Check sheet for the modelled part. Datum: model origin and axes. Units: mm. A direction names the side the tool comes from. Give positions to 0.01 mm unless a question says otherwise; leave off trailing zeros. Loops run counter-clockwise (first coordinate to the right, second up) from the corner with the lowest first, then second, coordinate; pieces in that order, holes last. Notation, with made-up numbers: (45.5, -23.75) - (73.5, -23.75) arc R15 cw to (73.5, 3.25) - close; hole circle Ø3 at (60.25, -30). An arc over 180 degrees is marked (long way). Use CSV: the item, a comma, the result in double quotes.
from build123d import *

# Parameters (mm, degrees)
F0_R     = 1
F0_R_2   = 1.5
F1_DEPTH = 0.5
F2_R     = 1
F2_R_2   = 2.2
F3_DEPTH = 1
F4_SIZE  = 0.99999
F5_R     = 1
F6_DEPTH = 1
F8_DEPTH = 1


# Not quite as in the source:
# - a fillet or chamfer is up to 0.001 mm smaller than in the source, because OpenCascade refuses the exact size


with BuildPart() as f1:
    # F0 (on Top) → F1 (new body)
    with BuildSketch(Plane.XY):
        with BuildLine():
            Line((-6.2, -5.1), (6.2, -5.1))
            ThreePointArc((6.2, -5.1), (8.3213203436, -4.2213203436), (9.2, -2.1))
            Line((9.2, -2.1), (9.2, 2.1))
            ThreePointArc((9.2, 2.1), (8.3213203436, 4.2213203436), (6.2, 5.1))
            Line((6.2, 5.1), (-6.2, 5.1))
            ThreePointArc((-6.2, 5.1), (-8.3213203436, 4.2213203436), (-9.2, 2.1))
            Line((-9.2, 2.1), (-9.2, -2.1))
            ThreePointArc((-9.2, -2.1), (-8.3213203436, -4.2213203436), (-6.2, -5.1))
        make_face()
        with Locations((-5.7, -2.2)):
            Circle(F0_R, mode=Mode.SUBTRACT)
        with Locations((5.7, -2.2)):
            Circle(F0_R, mode=Mode.SUBTRACT)
        with Locations((-5.7, 2.2)):
            Circle(F0_R, mode=Mode.SUBTRACT)
        Circle(F0_R_2, mode=Mode.SUBTRACT)
        with Locations((5.7, 2.2)):
            Circle(F0_R, mode=Mode.SUBTRACT)
    extrude(amount=F1_DEPTH)

    # F2 (on face) → F3 (join)
    with BuildSketch(Plane.XY.offset(0.5)):
        with BuildLine():
            ThreePointArc((-6.2, 5.1), (-8.3213203436, 4.2213203436), (-9.2, 2.1))
            Line((-9.2, 2.1), (-9.2, -2.1))
            ThreePointArc((-9.2, -2.1), (-8.3213203436, -4.2213203436), (-6.2, -5.1))
            Line((-6.2, -5.1), (6.2, -5.1))
            ThreePointArc((6.2, -5.1), (8.3213203436, -4.2213203436), (9.2, -2.1))
            Line((9.2, -2.1), (9.2, 2.1))
            ThreePointArc((9.2, 2.1), (8.3213203436, 4.2213203436), (6.2, 5.1))
            Line((6.2, 5.1), (-6.2, 5.1))
        make_face()
        with Locations((-5.7, -2.2)):
            Circle(F2_R, mode=Mode.SUBTRACT)
        Circle(F2_R_2, mode=Mode.SUBTRACT)
        with Locations((5.7, -2.2)):
            Circle(F2_R, mode=Mode.SUBTRACT)
        with Locations((-5.7, 2.2)):
            Circle(F2_R, mode=Mode.SUBTRACT)
        with Locations((5.7, 2.2)):
            Circle(F2_R, mode=Mode.SUBTRACT)
    extrude(amount=F3_DEPTH)

    # F4 (size 1 in the source; OpenCascade refuses exactly that, so slightly less here)
    f4_edges = [f1.edges().sort_by_distance(p)[0] for p in [
        (-2.2, 0, 1.5),
    ]]
    chamfer(f4_edges, length=F4_SIZE)

    # F5 (on face) → F6 (join)
    with BuildSketch(Plane.XY.offset(1.5)):
        with BuildLine():
            Line((6.2, 5.1), (-6.2, 5.1))
            ThreePointArc((-6.2, 5.1), (-8.3213203436, 4.2213203436), (-9.2, 2.1))
            Line((-9.2, 2.1), (-9.2, -2.1))
            ThreePointArc((-9.2, -2.1), (-8.3213203436, -4.2213203436), (-6.2, -5.1))
            Line((-6.2, -5.1), (6.2, -5.1))
            ThreePointArc((6.2, -5.1), (8.3213203436, -4.2213203436), (9.2, -2.1))
            Line((9.2, -2.1), (9.2, 2.1))
            ThreePointArc((9.2, 2.1), (8.3213203436, 4.2213203436), (6.2, 5.1))
        make_face()
        with Locations((-5.7, -2.2)):
            Circle(F5_R, mode=Mode.SUBTRACT)
        with BuildLine():
            ThreePointArc((3.5, -3), (3.3535533906, -3.3535533906), (3, -3.5))
            Line((3, -3.5), (-3, -3.5))
            ThreePointArc((-3, -3.5), (-3.3535533906, -3.3535533906), (-3.5, -3))
            Line((-3.5, -3), (-3.5, 3))
            ThreePointArc((-3.5, 3), (-3.3535533906, 3.3535533906), (-3, 3.5))
            Line((-3, 3.5), (3, 3.5))
            ThreePointArc((3, 3.5), (3.3535533906, 3.3535533906), (3.5, 3))
            Line((3.5, 3), (3.5, -3))
        make_face(mode=Mode.SUBTRACT)
        with Locations((5.7, -2.2)):
            Circle(F5_R, mode=Mode.SUBTRACT)
        with Locations((-5.7, 2.2)):
            Circle(F5_R, mode=Mode.SUBTRACT)
        with Locations((5.7, 2.2)):
            Circle(F5_R, mode=Mode.SUBTRACT)
    extrude(amount=F6_DEPTH)

    # F7 (on face) → F8 (join)
    with BuildSketch(Plane.XY.offset(2.5)):
        with BuildLine():
            ThreePointArc((6.2, -5.1), (8.3213203436, -4.2213203436), (9.2, -2.1))
            Line((9.2, -2.1), (9.2, 2.1))
            ThreePointArc((9.2, 2.1), (8.3213203436, 4.2213203436), (6.2, 5.1))
            Line((6.2, 5.1), (-6.2, 5.1))
            ThreePointArc((-6.2, 5.1), (-8.3213203436, 4.2213203436), (-9.2, 2.1))
            Line((-9.2, 2.1), (-9.2, -2.1))
            ThreePointArc((-9.2, -2.1), (-8.3213203436, -4.2213203436), (-6.2, -5.1))
            Line((-6.2, -5.1), (6.2, -5.1))
        make_face()
        with BuildLine():
            ThreePointArc((7.7, -3.5), (7.5535533906, -3.8535533906), (7.2, -4))
            Line((7.2, -4), (-7.2, -4))
            ThreePointArc((-7.2, -4), (-7.5535533906, -3.8535533906), (-7.7, -3.5))
            Line((-7.7, -3.5), (-7.7, 3.5))
            ThreePointArc((-7.7, 3.5), (-7.5535533906, 3.8535533906), (-7.2, 4))
            Line((-7.2, 4), (7.2, 4))
            ThreePointArc((7.2, 4), (7.5535533906, 3.8535533906), (7.7, 3.5))
            Line((7.7, 3.5), (7.7, -3.5))
        make_face(mode=Mode.SUBTRACT)
    extrude(amount=F8_DEPTH)


solid = f1.part
1. Sectioned sample at C-C, the plane x = 5.75. Record the boundary of the cut face in (y, z), and give its area (3 significant figures).
Completed:
outline,"(-5.1, 0) - (-3.2, 0) - (-3.2, 2.5) - (-4, 2.5) - (-4, 3.5) - (-5.1, 3.5) - close; (-1.2, 0) - (1.2, 0) - (1.2, 2.5) - (-1.2, 2.5) - close; (3.2, 0) - (5.1, 0) - (5.1, 3.5) - (4, 3.5) - (4, 2.5) - (3.2, 2.5) - close"
area,"17.7 mm²"
2. Release check for a two-part mould opening along X. For faces 3 (the face through (-8.3, 4.24, 1.73)), 4 (the face through (7.7, 0, 3)), 5 (the face through (2, 0, 0)), 6 (the face through (9.2, 0, 2)) record: released by +X, released by -X, zero draft, split by the parting line, or undercut.
Completed:
face 3,"released by -X"
face 4,"undercut"
face 5,"zero draft"
face 6,"released by +X"
3. Sectioned sample at D-D, the plane z = 1.8. Record the boundary of the cut face in (x, y).
Completed:
outline,"(-9.2, -2.1) arc R3 ccw to (-6.2, -5.1) - (6.2, -5.1) arc R3 ccw to (9.2, -2.1) - (9.2, 2.1) arc R3 ccw to (6.2, 5.1) - (-6.2, 5.1) arc R3 ccw to (-9.2, 2.1) - close; hole circle Ø2 at (-5.7, -2.2); hole circle Ø2 at (-5.7, 2.2); hole (-3.5, -3) arc R0.5 ccw to (-3, -3.5) - (3, -3.5) arc R0.5 ccw to (3.5, -3) - (3.5, 3) arc R0.5 ccw to (3, 3.5) - (-3, 3.5) arc R0.5 ccw to (-3.5, 3) - close; hole circle Ø2 at (5.7, -2.2); hole circle Ø2 at (5.7, 2.2)"
4. Set-up check for faces 1 (the face through (8.34, 4.2, 1.73)), 2 (the face through (0, -4, 3)): record each of +Z, -Z, +X, -X, +Y, -Y from which the full face is reachable in a straight line by a thin tool's end or side.
Completed:
face 1,"+Z, -Z, +X, +Y"
face 2,"+Z"
5. Go/stop test with flat-tipped pins: pin 1 Ø2.5 at (x, y) = (2.5, -1) entering from +Z; pin 2 Ø2.5 at (x, y) = (0, 0) entering from +Z; pin 3 Ø1.5 at (y, z) = (-4, 1) entering from +X; pin 4 Ø1.3 at (x, y) = (-1, 0.5) entering from +Z. Record where each tip stops, or that it passes through.
Completed:
pin 1,"stops at z = 2.5"
pin 2,"passes through"
pin 3,"stops at x = 8.97"
pin 4,"stops at z = 0.5"
6. Sectioned sample at B-B, the plane z = 0.95. Record the boundary of the cut face in (x, y), and give its area (3 significant figures).
Completed:
outline,"(-9.2, -2.1) arc R3 ccw to (-6.2, -5.1) - (6.2, -5.1) arc R3 ccw to (9.2, -2.1) - (9.2, 2.1) arc R3 ccw to (6.2, 5.1) - (-6.2, 5.1) arc R3 ccw to (-9.2, 2.1) - close; hole circle Ø2 at (-5.7, -2.2); hole circle Ø2 at (-5.7, 2.2); hole circle Ø5.3 at (0, 0); hole circle Ø2 at (5.7, -2.2); hole circle Ø2 at (5.7, 2.2)"
area,"145 mm²"
7. Scan lines: line 1 along Y through (x, z) = (5.7, 1.55); line 2 along Y through (x, z) = (-1, 1.95); line 3 along X through (y, z) = (1, 2.55). Record each from-to range of solid material in increasing order.
Completed:
line 1,"y = -5.1 to -3.2, -1.2 to 1.2, 3.2 to 5.1"
line 2,"y = -5.1 to -3.5, 3.5 to 5.1"
line 3,"x = -9.2 to -7.7, 7.7 to 9.2"
